```python
from build123d import *

# Parameters (mm, degrees)
SKETCH1_W           = 50
SKETCH1_H           = 85
BOSS_EXTRUDE1_DEPTH = 3.175
SKETCH3_W           = 37.782
SKETCH3_H           = 56.004
CUT_EXTRUDE1_DEPTH  = 99.666512176
FILLET2_R           = 1
FILLET3_R           = 5
SKETCH4_R           = 2
CUT_EXTRUDE2_DEPTH  = 99.666512176


with BuildPart() as part:
    # Sketch1 → Boss-Extrude1 (new body)
    with BuildSketch(Plane(origin=(0, 0, 0), x_dir=(1, 0, 0), z_dir=(0, 1, 0))):
        with Locations((25, 42.5)):
            Rectangle(SKETCH1_W, SKETCH1_H)
    extrude(amount=BOSS_EXTRUDE1_DEPTH)

    # Sketch3 → Cut-Extrude1 (cut, through all)
    with BuildSketch(Plane(origin=(0, 3.175, 0), x_dir=(1, 0, 0), z_dir=(0, 1, 0))):
        with Locations((25, 42.5)):
            Rectangle(SKETCH3_W, SKETCH3_H)
    extrude(amount=-CUT_EXTRUDE1_DEPTH, mode=Mode.SUBTRACT)

    # Fillet2
    fillet2_edges = [part.edges().sort_by_distance(p)[0] for p in [
        (6.109, 1.5875, -14.498),
        (6.109, 1.5875, -70.502),
        (43.891, 1.5875, -70.502),
        (43.891, 1.5875, -14.498),
    ]]
    fillet(fillet2_edges, radius=FILLET2_R)

    # Fillet3
    fillet3_edges = [part.edges().sort_by_distance(p)[0] for p in [
        (0, 1.5875, -85),
        (50, 1.5875, -85),
        (50, 1.5875, 0),
        (0, 1.5875, 0),
    ]]
    fillet(fillet3_edges, radius=FILLET3_R)

    # Sketch4 → Cut-Extrude2 (cut, through all)
    with BuildSketch(Plane(origin=(0, 3.175, 0), x_dir=(1, 0, 0), z_dir=(0, 1, 0))):
        with Locations(Location((5, 5, 0), (0, 0, 270))):
            Circle(SKETCH4_R)
        with Locations(Location((45, 5, 0), (0, 0, 270))):
            Circle(SKETCH4_R)
        with Locations(Location((45, 80, 0), (0, 0, 270))):
            Circle(SKETCH4_R)
        with Locations(Location((5, 80, 0), (0, 0, 270))):
            Circle(SKETCH4_R)
    extrude(amount=-CUT_EXTRUDE2_DEPTH, mode=Mode.SUBTRACT)


solid = part.part
```
Can you work these out from the model? Positions are in its coordinate system, mm. A direction names the side the tool comes from. Coordinates: 2 decimals unless noted, no trailing zeros. Write each loop counter-clockwise with the first axis right and the second up, starting at its lowest first coordinate (ties: lowest second). Pieces come first, ordered by that corner, then holes. Notation, with made-up numbers: M 63,-9.75 L 112,-9.75 A25 cw 112,7.25 Z; hole C 4,16.5 d5. An arc over 180 degrees is marked long. Write item = value, one per line. Start each with the question number.
Q1. Thinking about a two-plate mould opening in Z: for faces 1 (the face through (0, 2, -42)), 2 (the face through (1, 2, -2)), 3 (the face through (5.601, 1.61, -78.092)), which applies, released by +Z, released by -Z, zero draft, split by the parting line, or undercut?
Q2. If I drill on L1, parallel to X at y = 1.7, z = -80; L2, parallel to Z at x = 15, y = 0.3; L3, parallel to X at y = 2.65, z = -30, over which ranges is the centre line in solid material (lowest first)? Write a range as [from, to].
Q3. On a 3-axis mill with a long thin cutter (end or side, diameter ignored), from which of +Z, -Z, +X, -X, +Y, -Y can I reach the whole of each face in a straight line? I mean faces 4 (the face through (25, 2, -14.498)), 5 (the face through (50, 2, -42)). Say none if no direction works.
Q4. If we section it at C-C, the plane y = 2.25: Write out the boundary of the cut face in (x, z).
Q5. I'm going to push a flat-ended pin straight in: pin 1 (6.5 mm diameter, centred on x = 5, z = -5, fed in from -Y). Where does the tip first touch, or does it pass through?
Q6. If we section it at A-A, the plane x = 19: Write out the boundary of the cut face in (y, z) (3 decimals).
Q7. If we section it at B-B, the plane z = -67: Write out the boundary of the cut face in (x, y) (3 decimals).
Check sheet entries:
q1.face_1 = zero draft
q1.face_2 = released by +Z
q1.face_3 = undercut
q2.L1 = [0, 3], [7, 43], [47, 50]
q2.L2 = [-85, -70.5], [-14.5, 0]
q2.L3 = [0, 6.11], [43.89, 50]
q3.face_4 = +Y, -Y
q3.face_5 = +Z, -Z, +X, +Y, -Y
q4.outline = M 0,-80 A5 ccw 5,-85 L 45,-85 A5 ccw 50,-80 L 50,-5 A5 ccw 45,0 L 5,0 A5 ccw 0,-5 Z; hole C 5,-80 d4; hole C 5,-5 d4; hole M 6.11,-69.5 A1 ccw 7.11,-70.5 L 42.89,-70.5 A1 ccw 43.89,-69.5 L 43.89,-15.5 A1 ccw 42.89,-14.5 L 7.11,-14.5 A1 ccw 6.11,-15.5 Z; hole C 45,-80 d4; hole C 45,-5 d4
q5.pin_1 = 0
q6.outline = M 0,-85 L 3.175,-85 L 3.175,-70.502 L 0,-70.502 Z; M 0,-14.498 L 3.175,-14.498 L 3.175,0 L 0,0 Z
q7.outline = M 0,0 L 6.109,0 L 6.109,3.175 L 0,3.175 Z; M 43.891,0 L 50,0 L 50,3.175 L 43.891,3.175 Z
